Here's how the part is built. I have some questions about the finished solid (model axes, mm). A direction names the side the tool comes from. Give positions to 0.01 mm unless a question says otherwise; leave off trailing zeros. Loops run counter-clockwise (first coordinate to the right, second up) from the corner with the lowest first, then second, coordinate; pieces in that order, holes last. Notation, with made-up numbers: (68, -6.75) - (106, -6.75) arc R34 ccw to (106, 25.25) - close; hole circle Ø8 at (9.5, 42). An arc over 180 degrees is marked (long way). Use one line per item in the form item = value.
from build123d import *

# Parameters (mm, degrees)
BOSS_EXTRUDE1_DEPTH = 30
SKETCH3_W           = 60
SKETCH3_H           = 5
BOSS_EXTRUDE2_DEPTH = 20
SKETCH4_R           = 2.5
CUT_EXTRUDE1_DEPTH  = 126.034273701


with BuildPart() as part:
    # Sketch1 → Boss-Extrude1 (new, symmetric)
    with BuildSketch(Plane.XY):
        Polygon((0, 0), (0, 50), (37.64, 50), (37.64, 0), (32.64, 0), (32.64, 45), (5, 45), (5, 0), align=None)
    extrude(amount=BOSS_EXTRUDE1_DEPTH, both=True)

    # Sketch3 → Boss-Extrude2 (add)
    with BuildSketch(Plane.XZ):
        with Locations((67.64, 27.5)):
            Rectangle(SKETCH3_W, SKETCH3_H)
        with Locations((67.64, -27.5)):
            Rectangle(SKETCH3_W, SKETCH3_H)
    extrude(amount=-BOSS_EXTRUDE2_DEPTH)

    # Sketch4 → Cut-Extrude1 (cut, through all)
    with BuildSketch(Plane.XY.offset(30)):
        with Locations((62.64, 10)):
            Circle(SKETCH4_R)
    extrude(amount=-CUT_EXTRUDE1_DEPTH, mode=Mode.SUBTRACT)


solid = part.part
(1) If we section it at D-D (y = 26): List the corners of the cut face in (x, z) for me.
Geometry says:
outline = (0, -30) - (5, -30) - (5, 30) - (0, 30) - close; (32.64, -30) - (37.64, -30) - (37.64, 30) - (32.64, 30) - close
(2) For P1, Ø2.5, axis at x = 61.5, z = -27, coming from the +Y side; P2, Ø4, axis at x = 62.64, y = 10, coming from the -Z side; P3, Ø8.5, axis at x = 13.5, z = -14, coming from the -Y side, each with a flat end and sliding along its axis, tell me the tip position at first contact or that it passes through.
Geometry says:
P1 = 20
P2 = through
P3 = 45
(3) For faces 4 (the flat face through (67, 20, 28)), 5 (the flat face through (67, 10, -25)), 6 (the flat face through (5, 23, 0)), 7 (the flat face through (53, 16, -30)), which set-ups out of +Z, -Z, +X, -X, +Y, -Y let a thin tool reach every point of the face, with its end or its side?
Geometry says:
face_4 = +Z, -Z, +X, +Y
face_5 = +X, +Y, -Y
face_6 = +Z, -Z, -Y
face_7 = -Z, +X, -X, +Y, -Y
(4) If I drill on probe 1 along X at (y, z) = (25, 18.5); probe 2 along Y at (x, z) = (62.64, -28.6); probe 3 along Z at (x, y) = (93.5, 6), over which ranges is the centre line in solid material (lowest first)?
Geometry says:
probe_1 = 0 to 5, 32.64 to 37.64
probe_2 = 0 to 7.5, 12.5 to 20
probe_3 = -30 to -25, 25 to 30
(5) Thinking about a two-plate mould opening in Z: for faces 1 (the flat face through (37.64, 25, 0)), 2 (the cylindrical face through (65.025, 10.751, -27.465)), 3 (the flat face through (53, 16, 30)), which applies, pulls with the +Z half, pulls with the -Z half, needs draft (parallel to the pull), parting line crosses it, or undercut?
Geometry says:
face_1 = undercut
face_2 = needs draft
face_3 = pulls with the +Z half
(6) If we section it at A-A (x = 47.5): List the corners of the cut face in (y, z) for me, plus the area to 3 significant figures.
Geometry says:
outline = (0, -30) - (20, -30) - (20, -25) - (0, -25) - close; (0, 25) - (20, 25) - (20, 30) - (0, 30) - close
area = 200 mm²
(7) If we section it at B-B (y = 10): List the corners of the cut face in (x, z) for me, plus the area to 3 significant figures.
Geometry says:
outline = (0, -30) - (5, -30) - (5, 30) - (0, 30) - close; (32.64, -30) - (60.14, -30) - (60.14, -25) - (37.64, -25) - (37.64, 25) - (60.14, 25) - (60.14, 30) - (32.64, 30) - close; (65.14, -30) - (97.64, -30) - (97.64, -25) - (65.14, -25) - close; (65.14, 25) - (97.64, 25) - (97.64, 30) - (65.14, 30) - close
area = 1,150 mm²
(8) If we section it at C-C (z = -6): List the corners of the cut face in (x, y) for me, plus the area to 3 significant figures.
Geometry says:
outline = (0, 0) - (5, 0) - (5, 45) - (32.64, 45) - (32.64, 0) - (37.64, 0) - (37.64, 50) - (0, 50) - close
area = 638 mm²
